```python
from build123d import *

# Parameters (mm, degrees)
F0_W     = 3
F0_H     = 13.5
F1_DEPTH = 16.5
F2_R     = 1.25
F3_DEPTH = 4
F4_R     = 1.75
F5_DEPTH = 7.5
F6_R     = 0.5
F7_R     = 0.5
F8_R     = 0.5


with BuildPart() as f1:
    # F0 (on Front) → F1 (new body)
    with BuildSketch(Plane.XZ):
        with Locations((1.5, 9.75)):
            Rectangle(F0_W, F0_H)
        Polygon((3, 3), (0, 3), (0, 0), (16.5, 0), (16.5, 3), align=None)
    extrude(amount=F1_DEPTH)

    # F2 (on face) → F3 (join)
    with BuildSketch(Plane(origin=(0, 0, 0), x_dir=(1, 0, 0), z_dir=(0, 0, -1))):
        with Locations((8.25, 8.25)):
            Circle(F2_R)
    extrude(amount=F3_DEPTH)

    # F4 (on face) → F5 (join)
    with BuildSketch(Plane(origin=(0, 0, 0), x_dir=(0, -1, 0), z_dir=(-1, 0, 0))):
        with Locations((8.25, 8.25)):
            Circle(F4_R)
    extrude(amount=F5_DEPTH)

    # F6
    f6_edges = [f1.edges().sort_by_distance(p)[0] for p in [
        (7, -8.25, -4),
    ]]
    fillet(f6_edges, radius=F6_R)

    # F7
    f7_edges = [f1.edges().sort_by_distance(p)[0] for p in [
        (-7.5, -6.5, 8.25),
    ]]
    fillet(f7_edges, radius=F7_R)

    # F8
    f8_edges = [f1.edges().sort_by_distance(p)[0] for p in [
        (3, 0, 9.75),
        (3, -16.5, 9.75),
        (9.75, -16.5, 3),
        (9.75, 0, 3),
    ]]
    fillet(f8_edges, radius=F8_R)


solid = f1.part
```
Here's how the part is built. I have some questions about the finished solid (model axes, mm). A direction names the side the tool comes from. Give positions to 0.01 mm unless a question says otherwise; leave off trailing zeros. Write each loop counter-clockwise with the first axis right and the second up, starting at its lowest first coordinate (ties: lowest second). Pieces come first, ordered by that corner, then holes.
(1) Imagine slicing it at B-B, the plane z = 8.25. Write out the boundary of the cut face in (x, y).
Output values:
outline: (-7.5, -9.5) arc R0.5 ccw to (-7, -10) - (0, -10) - (0, -16.5) - (2.5, -16.5) arc R0.5 ccw to (3, -16) - (3, -0.5) arc R0.5 ccw to (2.5, 0) - (0, 0) - (0, -6.5) - (-7, -6.5) arc R0.5 ccw to (-7.5, -7) - close
(2) Imagine slicing it at D-D, the plane x = 14.5. Write out the boundary of the cut face in (y, z).
Output values:
outline: (-16.5, 0) - (0, 0) - (0, 2.5) arc R0.5 ccw to (-0.5, 3) - (-16, 3) arc R0.5 ccw to (-16.5, 2.5) - close
(3) Will these pins go through, and if not, where does the flat tip stop? pin 1 (3 mm diameter, centred on y = -9.5, z = 14, fed in from -X); pin 2 (7 mm diameter, centred on x = 10, y = -10.5, fed in from +Z); pin 3 (6 mm diameter, centred on x = 11, y = -4, fed in from -Z).
Output values:
pin 1: stops at x = 0
pin 2: stops at z = 3
pin 3: stops at z = 0
(4) Imagine slicing it at C-C, the plane y = -8.25. Write out the boundary of the cut face in (x, z).
Output values:
outline: (-7.5, 7) arc R0.5 ccw to (-7, 6.5) - (0, 6.5) - (0, 0) - (7, 0) - (7, -3.5) arc R0.5 ccw to (7.5, -4) - (9, -4) arc R0.5 ccw to (9.5, -3.5) - (9.5, 0) - (16.5, 0) - (16.5, 3) - (3, 3) - (3, 16.5) - (0, 16.5) - (0, 10) - (-7, 10) arc R0.5 ccw to (-7.5, 9.5) - close
(5) Imagine slicing it at A-A, the plane x = 8.25. Write out the boundary of the cut face in (y, z).
Output values:
outline: (-16.5, 0) - (-9.5, 0) - (-9.5, -3.5) arc R0.5 ccw to (-9, -4) - (-7.5, -4) arc R0.5 ccw to (-7, -3.5) - (-7, 0) - (0, 0) - (0, 2.5) arc R0.5 ccw to (-0.5, 3) - (-16, 3) arc R0.5 ccw to (-16.5, 2.5) - close
(6) If I drill on L1, parallel to X at y = -3.25, z = 9.75; L2, parallel to X at y = -15.5, z = 1.25, over which ranges is the centre line in solid material (lowest first)?
Output values:
L1: x = 0 to 3
L2: x = 0 to 16.5
(7) On a 3-axis mill with a long thin cutter (end or side, diameter ignored), from which of +Z, -Z, +X, -X, +Y, -Y can I reach the whole of each face in a straight line? I mean faces 1 (the face through (8, -8, -4)), 2 (the face through (7, -8.3, -1.7)), 3 (the face through (3, -8, 10)), 4 (the face through (-3.451, -9.919, 8.776)), 5 (the face through (2, 0, 5)). Say none if no direction works.
Output values:
face 1: -Z, +X, -X, +Y, -Y
face 2: -Z
face 3: +Z, +X, +Y, -Y
face 4: -X
face 5: +Z, -Z, +X, -X, +Y
